Build history of the part. All positions in model axes, mm. A direction names the side the tool comes from. Give positions to 0.01 mm unless a question says otherwise; leave off trailing zeros. Write each loop counter-clockwise with the first axis right and the second up, starting at its lowest first coordinate (ties: lowest second). Pieces come first, ordered by that corner, then holes.
from build123d import *

# Parameters (mm, degrees)
F1_DEPTH = 5
F2_DEPTH = 6
F3_DEPTH = 7
F4_DEPTH = 7


with BuildPart() as f1:
    # F0 (on Front) → F1 (new body)
    with BuildSketch(Plane.XZ):
        with BuildLine():
            Line((7, 11), (13, 11))
            ThreePointArc((13, 11), (17, 15), (13, 19))
            Line((13, 19), (7, 19))
            ThreePointArc((7, 19), (3, 15), (7, 11))
        make_face()
        with BuildLine():
            ThreePointArc((7, 13), (5, 15), (7, 17))
            Line((7, 17), (13, 17))
            ThreePointArc((13, 17), (15, 15), (13, 13))
            Line((13, 13), (7, 13))
        make_face(mode=Mode.SUBTRACT)
    extrude(amount=F1_DEPTH)



with BuildPart() as f1b:
    # F0 (on Front) → F1, piece 2 (new body)
    with BuildSketch(Plane.XZ):
        with BuildLine():
            ThreePointArc((63, 11), (67, 15), (63, 19))
            Line((63, 19), (57, 19))
            ThreePointArc((57, 19), (53, 15), (57, 11))
            Line((57, 11), (63, 11))
        make_face()
        with BuildLine():
            Line((57, 17), (63, 17))
            ThreePointArc((63, 17), (65, 15), (63, 13))
            Line((63, 13), (57, 13))
            ThreePointArc((57, 13), (55, 15), (57, 17))
        make_face(mode=Mode.SUBTRACT)
    extrude(amount=F1_DEPTH)


with BuildPart() as f2:
    # F0 (on Front) → F2 (new body)
    with BuildSketch(Plane.XZ):
        with BuildLine():
            Line((27, 15), (27, 0))
            Line((27, 0), (29, 0))
            Line((29, 0), (29, 15))
            ThreePointArc((29, 15), (35, 21), (41, 15))
            Line((41, 15), (41, 0))
            Line((41, 0), (43, 0))
            Line((43, 0), (43, 15))
            ThreePointArc((43, 15), (35, 23), (27, 15))
        make_face()
    extrude(amount=F2_DEPTH)


with BuildPart() as f1_1:
    add(f1.part)

    add(f1b.part)  # F3 merges F1b

    add(f2.part)  # F3 merges F2
    # F0 (on Front) → F3 (join)
    with BuildSketch(Plane.XZ):
        with BuildLine():
            Line((0, 30), (0, 0))
            Line((0, 0), (27, 0))
            Line((27, 0), (27, 15))
            ThreePointArc((27, 15), (35, 23), (43, 15))
            Line((43, 15), (43, 0))
            Line((43, 0), (70, 0))
            Line((70, 0), (70, 30))
            Line((70, 30), (0, 30))
        make_face()
        with BuildLine():
            ThreePointArc((13, 19), (17, 15), (13, 11))
            Line((13, 11), (7, 11))
            ThreePointArc((7, 11), (3, 15), (7, 19))
            Line((7, 19), (13, 19))
        make_face(mode=Mode.SUBTRACT)
        with BuildLine():
            Line((57, 19), (63, 19))
            ThreePointArc((63, 19), (67, 15), (63, 11))
            Line((63, 11), (57, 11))
            ThreePointArc((57, 11), (53, 15), (57, 19))
        make_face(mode=Mode.SUBTRACT)
    extrude(amount=F3_DEPTH)

    # F0 (on Front) → F4 (join)
    with BuildSketch(Plane.XZ):
        with BuildLine():
            Line((0, 30), (0, 0))
            Line((0, 0), (27, 0))
            Line((27, 0), (27, 15))
            ThreePointArc((27, 15), (35, 23), (43, 15))
            Line((43, 15), (43, 0))
            Line((43, 0), (70, 0))
            Line((70, 0), (70, 30))
            Line((70, 30), (0, 30))
        make_face()
        with BuildLine():
            ThreePointArc((13, 19), (17, 15), (13, 11))
            Line((13, 11), (7, 11))
            ThreePointArc((7, 11), (3, 15), (7, 19))
            Line((7, 19), (13, 19))
        make_face(mode=Mode.SUBTRACT)
        with BuildLine():
            Line((57, 19), (63, 19))
            ThreePointArc((63, 19), (67, 15), (63, 11))
            Line((63, 11), (57, 11))
            ThreePointArc((57, 11), (53, 15), (57, 19))
        make_face(mode=Mode.SUBTRACT)
    extrude(amount=F4_DEPTH)


solid = f1_1.part
(1) Saw through at B-B, the plane y = -2.5. List the corners of the cut face in (x, z).
(2) Saw through at C-C, the plane z = 9.25. List the corners of the cut face in (x, y), plus the area to 3 significant figures.
(3) Mould opens along X. For faces 4 (the face through (0, -3, 15)), 5 (the face through (55, -3, 0)), 6 (the face through (60, -2, 13)), 7 (the face through (65, -2, 15)) say: +X half, -X half, draft (parallel to the pull), parting line (faces both ways), or undercut.
(4) Probe line 1 (Z direction, x = 59.5, y = -2); line 2 (X direction, y = -5.25, z = 9); line 3 (X direction, y = -6.5, z = 2.5). List the from-to ranges inside material, lowest first.
(5) Drop flat-ended pins along their axis: pin 1 (2.5 mm diameter, centred on x = 12.5, z = 14.5, fed in from -Y); pin 2 (12 mm diameter, centred on x = 36, z = 15, fed in from -Y). Give the stop position or say it passes through.
(6) Saw through at A-A, the plane x = 9.5. List the corners of the cut face in (y, z), plus the area to 3 significant figures.
(7) 3-axis set-ups, long thin cutter, end or side, ignore diameter. For faces 1 (the face through (28, -6, 12)), 2 (the face through (60, -2, 17)), 3 (the face through (67, -6, 15)): which of +Z, -Z, +X, -X, +Y, -Y reach the whole face in a straight line?
(8) Saw through at D-D, the plane x = 35. List the corners of the cut face in (y, z), plus the area to 3 significant figures.
Computed values:
1. outline: (0, 0) - (29, 0) - (29, 15) arc R6 cw to (41, 15) - (41, 0) - (70, 0) - (70, 30) - (0, 30) - close; hole (7, 13) - (13, 13) arc R2 ccw to (13, 17) - (7, 17) arc R2 ccw to start; hole (57, 13) - (63, 13) arc R2 ccw to (63, 17) - (57, 17) arc R2 ccw to start
2. outline: (0, -7) - (27, -7) - (27, -6) - (29, -6) - (29, 0) - (0, 0) - close; (41, -6) - (43, -6) - (43, -7) - (70, -7) - (70, 0) - (41, 0) - close
2. area: 402 mm2
3. face 4: -X half
3. face 5: draft
3. face 6: undercut
3. face 7: undercut
4. line 1: z = 0 to 13, 17 to 30
4. line 2: x = 0 to 29, 41 to 70
4. line 3: x = 0 to 27, 43 to 70
5. pin 1: passes through
5. pin 2: stops at y = -6
6. outline: (-7, 0) - (0, 0) - (0, 13) - (-5, 13) - (-5, 11) - (-7, 11) - close; (-7, 19) - (-5, 19) - (-5, 17) - (0, 17) - (0, 30) - (-7, 30) - close
6. area: 174 mm2
7. face 1: -Z, -Y
7. face 2: +Y, -Y
7. face 3: -Y
8. outline: (-7, 23) - (-6, 23) - (-6, 21) - (0, 21) - (0, 30) - (-7, 30) - close
8. area: 61.0 mm2
